The model under review builds one solid part; all positions refer to its coordinate system, in mm. A direction names the side the tool comes from. Round coordinates to 2 decimals unless told otherwise and drop trailing zeros. Order: outer loops, then holes, each group sorted by start corner. A loop starts at its lowest first (then second) coordinate and runs counter-clockwise, first axis right, second up. Notation, with made-up numbers: M 81,-8.5 L 98,-8.5 A18 cw 98,10.5 Z; hole C 84,33 d11. An arc over 180 degrees is marked long. Use a Markdown table: item, result. Add a question column.
1. The part is to be moulded in two halves that separate along X. For faces 1 (the flat face through (115.926, -136, -187)), 2 (the flat face through (96, -116.536, -187)), 3 (the flat face through (-164.074, -136, -190)), say which applies: +X half, -X half, draft (parallel to the pull), parting line (faces both ways), or undercut.
2. To check wall thickness, follow probe 1 along Y at (x, z) = (93.5, -195); probe 2 along X at (y, z) = (133, -196); probe 3 along Z at (x, y) = (-159, 37). State the ranges of each line that lie inside material, in increasing order.
3. Consider section C-C on y = -79. State the section outline as (x, z) points.
4. Consider section A-A on z = -117.5. Count the separate pieces of the cut face and the enclosed holes in it, then the cut area to 3 significant figures.
5. For faces 4 (the flat face through (-184, -116.536, -190)), 5 (the flat face through (-184, -156.536, -190)), 6 (the flat face through (-164.074, 144, -187)), 7 (the flat face through (115.926, 144, -187)), 8 (the flat face through (96, 163.464, -187)), list the 3-axis set-ups (+Z, -Z, +X, -X, +Y, -Y) from which the entire face can be reached by the end or side of a thin tool; tool diameter is ignored.
6. Insertion check: P1, Ø1, axis at y = -124, z = -141.5, coming from the -X side; P2, Ø15, axis at x = 90.5, z = -125, coming from the -Y side; P3, Ø24, axis at y = -137, z = -125, coming from the +X side. Each pin has a flat end and moves straight along its axis. Give the tip position at first contact, or say it passes through.
7. Consider section B-B on x = -102. State the section outline as (y, z) points.
from build123d import *

# Parameters (mm, degrees)
F1_DEPTH = 20
F2_R     = 5
F3_W     = 40
F3_H     = 40
F4_DEPTH = 380
F5_F1_R  = 5
F5_F2_R  = 5
F6_R     = 5


with BuildPart() as f1:
    # F0 (on Top) → F1 (new body)
    with BuildSketch(Plane.XY):
        with BuildLine():
            Line((105.9260419756, 203.463898824), (-194.0739580244, 203.463898824))
            ThreePointArc((-194.0739580244, 203.463898824), (-229.4292970837, 188.8192378834), (-244.0739580244, 153.463898824))
            Line((-244.0739580244, 153.463898824), (-244.0739580244, -146.536101176))
            ThreePointArc((-244.0739580244, -146.536101176), (-229.4292970837, -181.8914402353), (-194.0739580244, -196.536101176))
            Line((-194.0739580244, -196.536101176), (105.9260419756, -196.536101176))
            ThreePointArc((105.9260419756, -196.536101176), (141.2813810349, -181.8914402353), (155.9260419756, -146.536101176))
            Line((155.9260419756, -146.536101176), (155.9260419756, 153.463898824))
            ThreePointArc((155.9260419756, 153.463898824), (141.2813810349, 188.8192378834), (105.9260419756, 203.463898824))
        make_face()
    extrude(amount=F1_DEPTH)

    # F2
    f2_edges = [f1.edges().sort_by_distance(p)[0] for p in [
        (-44.073958, 203.463899, 0),
        (-229.429297, 188.819238, 0),
        (-244.073958, 3.463899, 0),
        (-229.429297, -181.89144, 0),
        (-44.073958, -196.536101, 0),
        (141.281381, -181.89144, 0),
        (155.926042, 3.463899, 0),
        (141.281381, 188.819238, 0),
    ]]
    fillet(f2_edges, radius=F2_R)

    # F3 (on face) → F4 (join)
    with BuildSketch(Plane(origin=(0, 0, 0), x_dir=(1, 0, 0), z_dir=(0, 0, -1))):
        with Locations((95.9260419756, 136.536101176)):
            Rectangle(F3_W, F3_H)
        with Locations((95.9260419756, -143.463898824)):
            Rectangle(F3_W, F3_H)
        with Locations((-184.0739580244, -143.463898824)):
            Rectangle(F3_W, F3_H)
        with Locations((-184.0739580244, 136.536101176)):
            Rectangle(F3_W, F3_H)
    extrude(amount=F4_DEPTH)

    # F5: fillet of radius 5 on 20 edges, made by hand

    # F5_f1
    f5_f1_edges = [f1.edges().sort_by_distance(p)[0] for p in [
        (-164.0739580244, -156.536101176, -190),
        (-164.0739580244, -116.536101176, -190),
        (-204.0739580244, -156.536101176, -190),
        (-204.0739580244, -116.536101176, -190),
        (-204.0739580244, -136.536101176, -380),
        (75.9260419756, -156.536101176, -190),
        (115.9260419756, -156.536101176, -190),
        (115.9260419756, -116.536101176, -190),
        (75.9260419756, -116.536101176, -190),
        (115.9260419756, 123.463898824, -190),
        (115.9260419756, 163.463898824, -190),
        (75.9260419756, 163.463898824, -190),
        (75.9260419756, 123.463898824, -190),
        (-204.0739580244, 163.463898824, -190),
        (-204.0739580244, 123.463898824, -190),
        (-164.0739580244, 163.463898824, -190),
        (-164.0739580244, 123.463898824, -190),
        (-164.0739580244, 143.463898824, -380),
    ]]
    fillet(f5_f1_edges, radius=F5_F1_R)

    # F5_f2
    f5_f2_edges = [f1.edges().sort_by_distance(p)[0] for p in [
        (-204.0739580244, -136.536101176, 0),
        (-164.0739580244, 143.463898824, 0),
        (-165.5384241184, 161.99943273, 0),
        (-165.5384241184, 124.9283649181, 0),
        (-202.6094919303, -155.0716350819, 0),
        (-202.6094919303, -118.00056727, 0),
    ]]
    fillet(f5_f2_edges, radius=F5_F2_R)

    # F6
    f6_edges = [f1.edges().sort_by_distance(p)[0] for p in [
        (-44.073958, 203.463899, 20),
        (-229.429297, 188.819238, 20),
        (-244.073958, 3.463899, 20),
        (-229.429297, -181.89144, 20),
        (-44.073958, -196.536101, 20),
        (141.281381, -181.89144, 20),
        (155.926042, 3.463899, 20),
        (141.281381, 188.819238, 20),
    ]]
    fillet(f6_edges, radius=F6_R)


solid = f1.part
Answer block:
| question | item | result |
|---|---|---|
| 1 | face 1 | +X half |
| 1 | face 2 | draft |
| 1 | face 3 | undercut |
| 2 | probe 1 | -156.54 to -116.54, 123.46 to 163.46 |
| 2 | probe 2 | -204.07 to -164.07, 75.93 to 115.93 |
| 2 | probe 3 | 0 to 20 |
| 3 | outline | M -244.07,5 A5 ccw -239.07,0 L 150.93,0 A5 ccw 155.93,5 L 155.93,15 A5 ccw 150.93,20 L -239.07,20 A5 ccw -244.07,15 Z |
| 4 | separate pieces | 4 |
| 4 | enclosed holes | 0 |
| 4 | area | 6,310 mm^2 |
| 5 | face 4 | -Z, +X, -X |
| 5 | face 5 | -Z, +X, -X, -Y |
| 5 | face 6 | -Z, +Y, -Y |
| 5 | face 7 | -Z, +X, +Y, -Y |
| 5 | face 8 | -Z, +X, -X, +Y |
| 6 | P1 | x = -204.07 |
| 6 | P2 | y = -156.54 |
| 6 | P3 | x = 115.93 |
| 7 | outline | M -196.54,5 A5 ccw -191.54,0 L 198.46,0 A5 ccw 203.46,5 L 203.46,15 A5 ccw 198.46,20 L -191.54,20 A5 ccw -196.54,15 Z |
